from build123d import *

# Parameters (mm, degrees)
BOSS_EXTRUDE1_DEPTH  = 9.5
BOSS_EXTRUDE2_DEPTH  = 23
BOSS_EXTRUDE3_DEPTH  = 7.9
SKETCH5_R            = 11
SKETCH5_R_2          = 5
BOSS_EXTRUDE4_DEPTH  = 2
CUT_EXTRUDE1_START   = -3
SKETCH6_R            = 5
CUT_EXTRUDE1_DEPTH   = 3
SKETCH7_R            = 2.5
BOSS_EXTRUDE5_DEPTH  = 5
SKETCH8_R            = 2.5
BOSS_EXTRUDE6_DEPTH  = 23.3
CUT_EXTRUDE2_DEPTH   = 17
SKETCH10_W           = 26
SKETCH10_H           = 14.120419237
BOSS_EXTRUDE7_DEPTH  = 0.01
SKETCH11_W           = 3.2
SKETCH11_H           = 16
BOSS_EXTRUDE8_DEPTH  = 3.9
BOSS_EXTRUDE9_DEPTH  = 5.6
SKETCH13_W           = 0.930512921
SKETCH13_H           = 15
BOSS_EXTRUDE10_DEPTH = 3.9
SKETCH14_W           = 0.930512921
SKETCH14_H           = 15
BOSS_EXTRUDE11_DEPTH = 0.1
BOSS_EXTRUDE12_DEPTH = 5
SKETCH16_R           = 0.25
BOSS_EXTRUDE13_DEPTH = 5
SKETCH17_R           = 1.5
CUT_EXTRUDE3_DEPTH   = 5.5
SKETCH18_R           = 3.25
CUT_EXTRUDE4_DEPTH   = 3
CUT_EXTRUDE5_START   = -4
SKETCH20_R           = 1.5
CUT_EXTRUDE5_DEPTH   = 4
SKETCH21_R           = 4.5
CUT_EXTRUDE6_DEPTH   = 4


with BuildPart() as part:
    # Sketch1 → Boss-Extrude1 (new body)
    with BuildSketch(Plane.XY):
        Polygon((-17, 21), (-21, 17), (-21, -17), (-17, -21), (17, -21), (21, -17), (21, 17), (17, 21), align=None)
    extrude(amount=BOSS_EXTRUDE1_DEPTH)

    # Sketch2 → Boss-Extrude2 (add)
    with BuildSketch(Plane.XY.offset(9.5)):
        Polygon((14, 21.15), (21.15, 14), (21.15, -14), (14, -21.15), (-14, -21.15), (-21.15, -14), (-21.15, 14), (-14, 21.15), align=None)
    extrude(amount=BOSS_EXTRUDE2_DEPTH)

    # Sketch3 → Boss-Extrude3 (add)
    with BuildSketch(Plane.XY.offset(32.5)):
        Polygon((-17, 21), (17, 21), (21, 17), (21, -17), (17, -21), (-17, -21), (-21, -17), (-21, 17), align=None)
    extrude(amount=BOSS_EXTRUDE3_DEPTH)

    # Sketch5 → Boss-Extrude4 (add)
    with BuildSketch(Plane.XY.offset(40.4)):
        with Locations(Location((0, 0, 0), (0, 0, 180))):
            Circle(SKETCH5_R)
        Circle(SKETCH5_R_2, mode=Mode.SUBTRACT)
    extrude(amount=BOSS_EXTRUDE4_DEPTH)

    # Sketch6 → Cut-Extrude1 (cut)
    with BuildSketch(Plane.XY.offset(40.4).offset(CUT_EXTRUDE1_START)):
        Circle(SKETCH6_R)
    extrude(amount=CUT_EXTRUDE1_DEPTH, mode=Mode.SUBTRACT)

    # Sketch7 → Boss-Extrude5 (add)
    with BuildSketch(Plane.XY.offset(37.4)):
        with Locations(Location((0, 0, 0), (0, 0, 180))):
            Circle(SKETCH7_R)
    extrude(amount=BOSS_EXTRUDE5_DEPTH)

    # Sketch8 → Boss-Extrude6 (add)
    with BuildSketch(Plane.XY.offset(42.4)):
        with Locations(Location((0, 0, 0), (0, 0, 180))):
            Circle(SKETCH8_R)
    extrude(amount=BOSS_EXTRUDE6_DEPTH)

    # Sketch9 → Cut-Extrude2 (cut)
    with BuildSketch(Plane.XY.offset(65.7)):
        Polygon((-2.316645086, 2.1), (3.697939095, 2.1), (-0.123554347, 3.991048302), align=None)
    extrude(amount=-CUT_EXTRUDE2_DEPTH, mode=Mode.SUBTRACT)

    # Sketch10 → Boss-Extrude7 (add)
    with BuildSketch(Plane(origin=(0, 21.15, 0), x_dir=(1, 0, 0), z_dir=(0, 1, 0))):
        with Locations((0, -20.751085576)):
            Rectangle(SKETCH10_W, SKETCH10_H)
    extrude(amount=BOSS_EXTRUDE7_DEPTH)

    # Sketch11 → Boss-Extrude8 (add)
    with BuildSketch(Plane(origin=(21, 0, 0), x_dir=(0, 0, -1), z_dir=(1, 0, 0))):
        with Locations((-1.645589959, 0)):
            Rectangle(SKETCH11_W, SKETCH11_H)
    extrude(amount=BOSS_EXTRUDE8_DEPTH)

    # Sketch12 → Boss-Extrude9 (add)
    with BuildSketch(Plane(origin=(21, 0, 0), x_dir=(0, 0, -1), z_dir=(1, 0, 0))):
        Polygon((-9.5, 7.2), (-4.97610288, 7.2), (-4.97610288, -7.2), (-9.5, -7.2), (-9.5, -8), (-4.17610288, -8), (-4.17610288, -7.2), (-4.17610288, 7.2), (-4.17610288, 8), (-9.5, 8), align=None)
    extrude(amount=BOSS_EXTRUDE9_DEPTH)

    # Sketch13 → Boss-Extrude10 (add)
    with BuildSketch(Plane(origin=(21, 0, 0), x_dir=(0, 0, -1), z_dir=(1, 0, 0))):
        with Locations((-3.71084642, 0)):
            Rectangle(SKETCH13_W, SKETCH13_H)
    extrude(amount=BOSS_EXTRUDE10_DEPTH)

    # Sketch14 → Boss-Extrude11 (add)
    with BuildSketch(Plane(origin=(24.9, 0, 0), x_dir=(0, 0, -1), z_dir=(1, 0, 0))):
        with Locations((-3.71084642, 0)):
            Rectangle(SKETCH14_W, SKETCH14_H)
    extrude(amount=BOSS_EXTRUDE11_DEPTH)

    # Sketch15 → Boss-Extrude12 (add)
    with BuildSketch(Plane(origin=(21, 0, 0), x_dir=(0, 0, -1), z_dir=(1, 0, 0))):
        Polygon((-5.97610288, 6.2), (-9, 6.2), (-9, 4), (-9.5, 4), (-9.5, 6.7), (-9, 6.7), (-5.47610288, 6.7), (-5.47610288, -6.7), (-9, -6.7), (-9.5, -6.7), (-9.5, -4), (-9, -4), (-9, -6.2), (-5.97610288, -6.2), align=None)
    extrude(amount=BOSS_EXTRUDE12_DEPTH)

    # Sketch16 → Boss-Extrude13 (add)
    with BuildSketch(Plane(origin=(21, 0, 0), x_dir=(0, 0, -1), z_dir=(1, 0, 0))):
        with Locations(Location((-7.48805144, 5, 0), (0, 0, 270))):
            Circle(SKETCH16_R)
        with Locations(Location((-7.48805144, 3, 0), (0, 0, 270))):
            Circle(SKETCH16_R)
        with Locations(Location((-7.48805144, 1, 0), (0, 0, 270))):
            Circle(SKETCH16_R)
        with Locations(Location((-7.48805144, -1, 0), (0, 0, 270))):
            Circle(SKETCH16_R)
        with Locations(Location((-7.48805144, -3, 0), (0, 0, 270))):
            Circle(SKETCH16_R)
        with Locations(Location((-7.48805144, -5, 0), (0, 0, 270))):
            Circle(SKETCH16_R)
    extrude(amount=BOSS_EXTRUDE13_DEPTH)

    # Sketch17 → Cut-Extrude3 (cut)
    with BuildSketch(Plane.XY.offset(40.4)):
        with Locations((-15.5, 15.5)):
            Circle(SKETCH17_R)
        with Locations((15.5, 15.5)):
            Circle(SKETCH17_R)
        with Locations((15.5, -15.5)):
            Circle(SKETCH17_R)
        with Locations((-15.5, -15.5)):
            Circle(SKETCH17_R)
    extrude(amount=-CUT_EXTRUDE3_DEPTH, mode=Mode.SUBTRACT)

    # Sketch18 → Cut-Extrude4 (cut)
    with BuildSketch(Plane(origin=(0, 0, 0), x_dir=(-1, 0, 0), z_dir=(0, 0, -1))):
        with Locations((-15.5, 15.5)):
            Circle(SKETCH18_R)
        with Locations((15.5, 15.5)):
            Circle(SKETCH18_R)
        with Locations((15.5, -15.5)):
            Circle(SKETCH18_R)
        with Locations((-15.5, -15.5)):
            Circle(SKETCH18_R)
    extrude(amount=-CUT_EXTRUDE4_DEPTH, mode=Mode.SUBTRACT)

    # Sketch20 → Cut-Extrude5 (cut)
    with BuildSketch(Plane(origin=(0, 0, 3), x_dir=(-1, 0, 0), z_dir=(0, 0, -1)).offset(CUT_EXTRUDE5_START)):
        with Locations(Location((-15.5, 15.5, 0), (0, 0, 180))):
            Circle(SKETCH20_R)
        with Locations(Location((15.5, 15.5, 0), (0, 0, 180))):
            Circle(SKETCH20_R)
        with Locations(Location((-15.5, -15.5, 0), (0, 0, 180))):
            Circle(SKETCH20_R)
        with Locations(Location((15.5, -15.5, 0), (0, 0, 180))):
            Circle(SKETCH20_R)
    extrude(amount=CUT_EXTRUDE5_DEPTH, mode=Mode.SUBTRACT)

    # Sketch21 → Cut-Extrude6 (cut)
    with BuildSketch(Plane(origin=(0, 0, 0), x_dir=(-1, 0, 0), z_dir=(0, 0, -1))):
        Circle(SKETCH21_R)
    extrude(amount=-CUT_EXTRUDE6_DEPTH, mode=Mode.SUBTRACT)


solid = part.part
Geometry check sheet. Reference: the model listing, model coordinates, mm. A direction names the side the tool comes from. Round coordinates to 2 decimals unless told otherwise and drop trailing zeros. Loops run counter-clockwise (first coordinate to the right, second up) from the corner with the lowest first, then second, coordinate; pieces in that order, holes last.
Item 1: Mould release check, pull along Y, two halves, no side actions. Record for faces 5 (the cylindrical face through (-17, -15.57, 5.03)), 6 (the flat face through (23, 8, 2)), 7 (the flat face through (24, 5, 9.5)), 8 (the cylindrical face through (-17, -15.43, 37.69)): pulls with the +Y half, pulls with the -Y half, needs draft (parallel to the pull), parting line crosses it, or undercut.
Item 2: Thickness scan on line 1 (X direction, y = -15.5, z = 3.9); line 2 (Y direction, x = 0, z = 40.05). Record the ranges inside material, lowest first.
Item 3: Cross-section at A-A on z = 34. Record the boundary of the cut face in (x, y), then the cut area to 3 significant figures.
Item 4: Cross-section at B-B on x = 20. Record the boundary of the cut face in (y, z), then the cut area to 3 significant figures.
Item 5: Access from +Z, -Z, +X, -X, +Y, -Y to the whole of each face (thin tool, end or side, straight path). Record for faces 1 (the flat face through (15, 15, 7)), 2 (the flat face through (0, -21, 5)), 3 (the flat face through (17.63, -17.52, 20.84)), 4 (the flat face through (-16, 16, 34.9)).
Item 6: Gauge pin test, flat ends, axial feed: pin 1 (12 mm diameter, centred on y = -3, z = 30, fed in from +X); pin 2 (2 mm diameter, centred on x = -0.5, y = 7, fed in from -Z); pin 3 (6 mm diameter, centred on x = -6, y = 9.5, fed in from +Z); pin 4 (2 mm diameter, centred on y = 3, z = 34, fed in from -X). Record the tip position at first contact, or that the pin passes through.
Answer sheet:
1. face 5: undercut
1. face 6: pulls with the +Y half
1. face 7: needs draft
1. face 8: undercut
2. line 1: x = -21 to -17, -14 to 14, 17 to 21
2. line 2: y = -21 to -5, -2.5 to 2.5, 5 to 21
3. outline: (-21, -17) - (-17, -21) - (17, -21) - (21, -17) - (21, 17) - (17, 21) - (-17, 21) - (-21, 17) - close
3. area: 1,730 mm2
4. outline: (-18, 0) - (18, 0) - (18, 9.5) - (15.15, 9.5) - (15.15, 32.5) - (18, 32.5) - (18, 40.4) - (-18, 40.4) - (-18, 32.5) - (-15.15, 32.5) - (-15.15, 9.5) - (-18, 9.5) - close
4. area: 1,320 mm2
5. face 1: -Z
5. face 2: -Z, +X, -X, -Y
5. face 3: +X, -Y
5. face 4: +Z
6. pin 1: stops at x = 21.15
6. pin 2: stops at z = 0
6. pin 3: stops at z = 42.4
6. pin 4: stops at x = -21
